from build123d import *

# Parameters (mm, degrees)
BOSS_EXTRUDE1_DEPTH = 7
FILLET1_R           = 2.5
SKETCH2_R           = 5.410546581
BOSS_EXTRUDE2_DEPTH = 7
FILLET2_R           = 2.5
SKETCH3_R           = 3
CUT_EXTRUDE1_DEPTH  = 16
SKETCH4_R           = 63
SKETCH4_R_2         = 61
CUT_EXTRUDE2_DEPTH  = 28


with BuildPart() as part:
    # Sketch1 → Boss-Extrude1 (new body)
    with BuildSketch(Plane(origin=(0, 0, 0), x_dir=(1, 0, 0), z_dir=(0, 1, 0))):
        Polygon((-6.297256143, 55.195428384), (0.702743857, 55.195428384), (33.702743857, 55.195428384), (33.702743857, 48.195428384), (0.702743857, 48.195428384), (0.702743857, -24.804571616), (-6.297256143, -24.804571616), align=None)
    extrude(amount=BOSS_EXTRUDE1_DEPTH)

    # Fillet1
    fillet1_edges = [part.edges().sort_by_distance(p)[0] for p in [
        (-6.297256143, 7, -15.195428384),
        (0.702743857, 7, -11.695428384),
        (-6.297256143, 0, -15.195428384),
        (0.702743857, 0, -11.695428384),
    ]]
    fillet(fillet1_edges, radius=FILLET1_R)

    # Sketch2 → Boss-Extrude2 (add)
    with BuildSketch(Plane(origin=(0, 0, -55.195428384), x_dir=(-1, 0, 0), z_dir=(0, 0, -1))):
        with Locations((-31.362766576, 3.435192577)):
            Circle(SKETCH2_R)
    extrude(amount=-BOSS_EXTRUDE2_DEPTH)

    # Fillet2
    fillet2_edges = [part.edges().sort_by_distance(p)[0] for p in [
        (27.182639034, 0, -51.695428384),
        (27.2926115, 7, -51.695428384),
    ]]
    fillet(fillet2_edges, radius=FILLET2_R)

    # Sketch3 → Cut-Extrude1 (cut)
    with BuildSketch(Plane(origin=(0, 0, -55.195428384), x_dir=(-1, 0, 0), z_dir=(0, 0, -1))):
        with Locations((-31.229894895, 3.460516579)):
            Circle(SKETCH3_R)
    extrude(amount=-CUT_EXTRUDE1_DEPTH, mode=Mode.SUBTRACT)

    # Sketch4 → Cut-Extrude2 (cut)
    with BuildSketch(Plane.XY.offset(24.804571616)):
        with Locations((58.808648779, 1.743015897)):
            Circle(SKETCH4_R)
        with Locations((58.808648779, 1.743015897)):
            Circle(SKETCH4_R_2, mode=Mode.SUBTRACT)
    extrude(amount=-CUT_EXTRUDE2_DEPTH, mode=Mode.SUBTRACT)


solid = part.part
Design review of the part built by this model. Coordinates are the model's own, in mm. A direction names the side the tool comes from. Give positions to 0.01 mm unless a question says otherwise; leave off trailing zeros. Loops run counter-clockwise (first coordinate to the right, second up) from the corner with the lowest first, then second, coordinate; pieces in that order, holes last. Notation, with made-up numbers: (44, -38.5) - (54, -38.5) arc R13 cw to (54, -18.5) - close; hole circle Ø10 at (26.5, 0). An arc over 180 degrees is marked (long way). Write item = value, one per line.
1) To check wall thickness, follow line 1 (Z direction, x = 14.5, y = 1.75); line 2 (Y direction, x = 25.5, z = -50.5); line 3 (X direction, y = 4, z = 0.5). State the ranges of each line that lie inside material, in increasing order.
Result sheet:
line_1 = -55.2 to -48.2
line_2 = 0 to 7
line_3 = -6.3 to -4.15, -2.15 to 0.7
2) Take a section at A-A on y = 1.5. State the section outline as (x, z) points, and give its area (3 significant figures).
Result sheet:
outline = (-6.09, -55.2) - (28.96, -55.2) - (28.96, -48.2) - (0.49, -48.2) - (0.49, 24.8) - (-2.19, 24.8) - (-2.19, -3.2) - (-4.19, -3.2) - (-4.19, 24.8) - (-6.09, 24.8) - close; (33.5, -55.2) - (36.42, -55.2) - (36.42, -48.2) - (33.5, -48.2) - close
area = 690 mm2
3) Take a section at C-C on z = 12. State the section outline as (x, y) points, and give its area (3 significant figures).
Result sheet:
outline = (-6.3, 2.5) arc R2.5 ccw to (-4.17, 0.03) arc R63 cw to (-3.97, 6.99) arc R2.5 ccw to (-6.3, 4.5) - close; (-2.17, 0) - (-1.8, 0) arc R2.5 ccw to (0.7, 2.5) - (0.7, 4.5) arc R2.5 ccw to (-1.8, 7) - (-1.96, 7) arc R61 ccw to start
area = 29.6 mm2
4) Draft analysis for pull direction X (two halves, no side actions). For faces 3 (the face through (-6.297, 3, -15)), 4 (the face through (0.703, 3, -12)), 5 (the face through (-4.165, 3.562, 11.001)), state which applies: +X half, -X half, draft (parallel to the pull), parting line (faces both ways), or undercut.
Result sheet:
face_3 = -X half
face_4 = +X half
face_5 = undercut
5) Take a section at B-B on z = -34.5. State the section outline as (x, y) points.
Result sheet:
outline = (-6.3, 2.5) arc R2.5 ccw to (-3.8, 0) - (-1.8, 0) arc R2.5 ccw to (0.7, 2.5) - (0.7, 4.5) arc R2.5 ccw to (-1.8, 7) - (-3.8, 7) arc R2.5 ccw to (-6.3, 4.5) - close
6) Tool access review of faces 1 (the face through (-2, 7, -42)), 2 (the face through (-0.01, 0.75, -11.18)): name each direction out of +Z, -Z, +X, -X, +Y, -Y from which nothing blocks a thin tool from reaching the whole face with its end or side.
Result sheet:
face_1 = +Z, -Z, -X, +Y
face_2 = +Z, +X, -Y
7) Clearance check with flat-ended pins moving along their axes: pin 1 Ø2 at (x, y) = (27, 2.5) entering from +Z; pin 2 Ø0.7 at (x, y) = (-2.5, 5) entering from +Z; pin 3 Ø2 at (y, z) = (3, -12.5) entering from +X. State where each tip first meets the part, or that it passes through.
Result sheet:
pin_1 = -48.2
pin_2 = -3.2
pin_3 = 0.7
8) Take a section at D-D on y = 5.5. State the section outline as (x, z) points.
Result sheet:
outline = (-6.09, -55.2) - (29.03, -55.2) - (29.03, -48.2) - (0.49, -48.2) - (0.49, 24.8) - (-2.08, 24.8) - (-2.08, -3.2) - (-4.08, -3.2) - (-4.08, 24.8) - (-6.09, 24.8) - close; (33.43, -55.2) - (36.36, -55.2) - (36.36, -48.2) - (33.43, -48.2) - close
